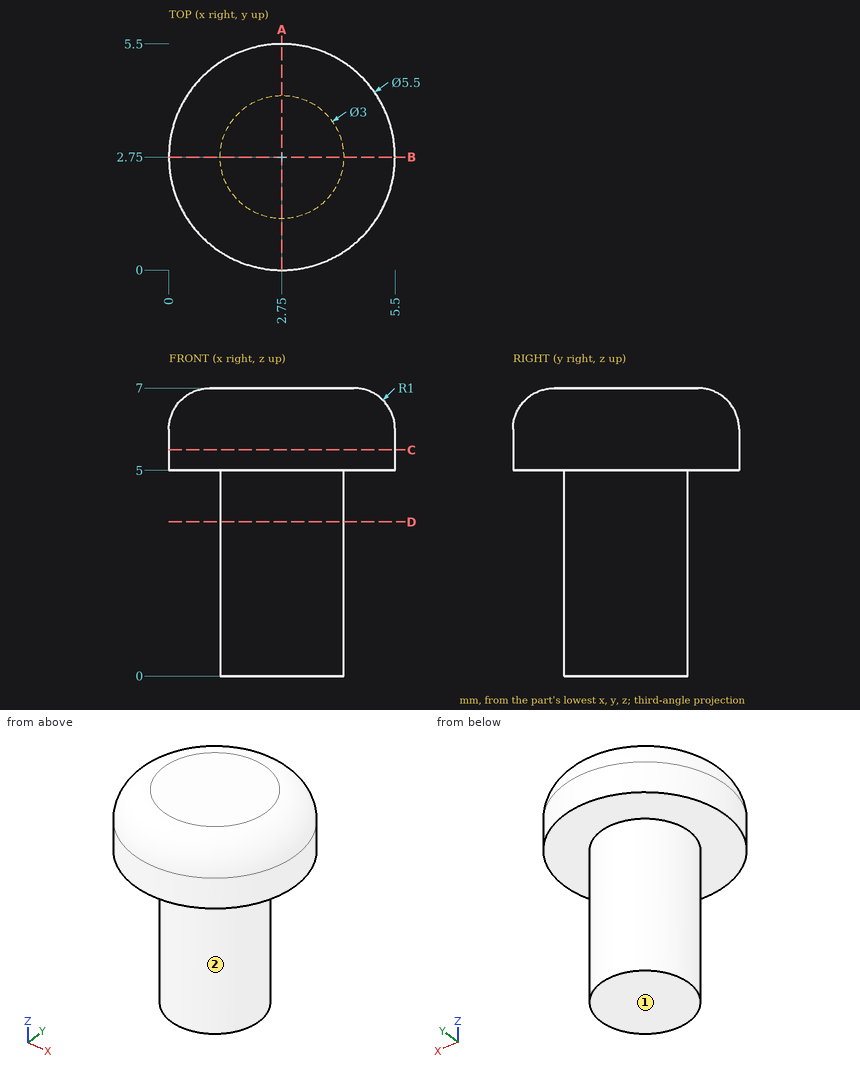
Design review of the part shown in the three views and the two pictorial views. Dimensions are in mm from the part's minimum x, y and z. A direction names the side the tool comes from. Coordinates: 2 decimals unless noted, no trailing zeros. Loops run counter-clockwise (first coordinate to the right, second up) from the corner with the lowest first, then second, coordinate; pieces in that order, holes last.
Q1. Tool access review of the marked faces 1 and 2: name each direction out of +Z, -Z, +X, -X, +Y, -Y from which nothing blocks a thin tool from reaching the whole face with its end or side.
Reported:
face 1: -Z, +X, -X, +Y, -Y
face 2: -Z
Q2. We need section A-A on x = 2.75. State the section outline as (y, z) points, and give its area (3 significant figures).
Reported:
outline: (0, 5) - (1.25, 5) - (1.25, 0) - (4.25, 0) - (4.25, 5) - (5.5, 5) - (5.5, 6) arc R1 ccw to (4.5, 7) - (1, 7) arc R1 ccw to (0, 6) - close
area: 25.6 mm2
Q3. We need section C-C on z = 5.5. State the section outline as (x, y) points.
Reported:
outline: circle Ø5.5 at (2.75, 2.75)
Q4. We need section D-D on z = 3.75. State the section outline as (x, y) points, and give its area (3 significant figures).
Reported:
outline: circle Ø3 at (2.75, 2.75)
area: 7.07 mm2
Q5. For pin 1 (1.5 mm diameter, centred on y = 2, z = 2.5, fed in from +X), flat-tipped, find the tip position at first contact; note if it passes through.
Reported:
pin 1: stops at x = 4.25
Q6. To check wall thickness, follow line 1 (Z direction, x = 1.2, y = 2.1); line 2 (X direction, y = 3.5, z = 6.5); line 3 (Y direction, x = 2.4, z = 5.75). State the ranges of each line that lie inside material, in increasing order.
Reported:
line 1: z = 5 to 7
line 2: x = 0.24 to 5.26
line 3: y = 0.02 to 5.48
